from build123d import *

# Parameters (mm, degrees)
BOSS_EXTRUDE1_DEPTH      = 3.175
BOSS_EXTRUDE1_DEPTH_BACK = 19.05
SKETCH2_R                = 6.35
CUT_EXTRUDE1_DEPTH       = 41.348741461
CUT_EXTRUDE1_DEPTH_BACK  = 41.348741461
SKETCH3_R                = 0.79375
FILLET1_R                = 3.175
CHAMFER1_SIZE            = 1.27


with BuildPart() as part:
    # Sketch1 → Revolve1 (revolve)
    with BuildSketch(Plane.XY, mode=Mode.PRIVATE) as revolve1_sk:
        with BuildLine():
            Line((-1.5875, -19.05), (-1.5875, -23.8125))
            Line((-1.5875, -23.8125), (-3.175, -23.8125))
            Line((-3.175, -23.8125), (-3.175, 0))
            Line((-3.175, 0), (3.175, 0))
            Line((3.175, 0), (3.175, -23.8125))
            Line((3.175, -23.8125), (1.5875, -23.8125))
            Line((1.5875, -23.8125), (1.5875, -19.05))
            ThreePointArc((1.5875, -19.05), (0, -17.4625), (-1.5875, -19.05))
        make_face()
    revolve(revolve1_sk.sketch.rotate(Axis((-3.175, 0, 0), (1, 0, 0)), 270), axis=Axis((-3.175, 0, 0), (1, 0, 0)))

    # Sketch2 → Boss-Extrude1 (add, two sides: drawn at the far end of the back side and taken through both)
    with BuildSketch(Plane.ZY.offset(3.175).offset(-BOSS_EXTRUDE1_DEPTH_BACK)):
        Circle(SKETCH2_R)
    extrude(amount=BOSS_EXTRUDE1_DEPTH + BOSS_EXTRUDE1_DEPTH_BACK)

    # Sketch3 → Cut-Extrude1 (cut, two sides: drawn at the far end of the back side and taken through both)
    with BuildSketch(Plane.ZY.offset(6.35).offset(-CUT_EXTRUDE1_DEPTH_BACK)):
        Circle(SKETCH3_R)
    extrude(amount=CUT_EXTRUDE1_DEPTH + CUT_EXTRUDE1_DEPTH_BACK, mode=Mode.SUBTRACT)

    # Fillet1
    fillet1_edges = [part.edges().sort_by_distance(p)[0] for p in [
        (-3.175, 0, -6.35),
        (3.175, 0, -6.35),
    ]]
    fillet(fillet1_edges, radius=FILLET1_R - 0.0001)  # a hair under: the kernel refuses the full size

    # Chamfer1
    chamfer1_edges = [part.edges().sort_by_distance(p)[0] for p in [
        (-1.5875, 0, -23.8125),
        (1.5875, 0, -23.8125),
    ]]
    chamfer(chamfer1_edges, length=CHAMFER1_SIZE)


solid = part.part
The listing builds one solid part. Answer for the finished solid, in the listing's coordinates (mm). A direction names the side the tool comes from. Round coordinates to 2 decimals unless told otherwise and drop trailing zeros. Order: outer loops, then holes, each group sorted by start corner. A loop starts at its lowest first (then second) coordinate and runs counter-clockwise, first axis right, second up. Notation, with made-up numbers: (66.25, 63.5) -> (103.25, 63.5) arc R19 ccw to (103.25, 99.5) -> close; hole circle Ø1 at (56.5, 25). An arc over 180 degrees is marked (long way). Write each question's results on one line, items separated by ' | '. Start each with the question number.
Q1. Which of the six approach directions +Z, -Z, +X, -X, +Y, -Y give full straight-line access (tool end or side, diameter ignored) to faces 1 (the flat face through (1.587, -17, -10)), 2 (the flat face through (3.175, 0, -10)), 3 (the flat face through (15.875, 0, 1)), 4 (the flat face through (-3.175, 0, 10))?
Q2. Find section D-D (x = 5.5). Determine the outline of the cut face in (y, z).
Q3. The mould has two halves that part along Z. Classify faces 5 (the cylindrical face through (4.918, -0.775, -0.172)), 6 (the flat face through (-6.35, 0, 1)), 7 (the cylindrical face through (3.014, 23.246, -5.162)): pulls with the +Z half, pulls with the -Z half, needs draft (parallel to the pull), parting line crosses it, or undercut.
Q4. Straight lines are drawn through the part: probe 1 along Z at (x, y) = (11, 0); probe 2 along X at (y, z) = (-13.5, 14) (1 decimal). For each, find the intervals that lie inside material, in ascending order. Write a range as from..to.
Q5. Find section C-C (x = 10.25). Determine the outline of the cut face in (y, z).
Q6. Each of these flat-tipped pins is pushed along its axis until it touches: pin 1 (12 mm diameter, centred on y = -15, z = -10, fed in from +X) (3 decimals); pin 2 (3 mm diameter, centred on y = 14.5, z = 3.5, fed in from -X) (3 decimals); pin 3 (8 mm diameter, centred on x = 4.5, y = -10, fed in from -Z); pin 4 (1.3 mm diameter, centred on y = 0, z = 0, fed in from -X). Where does it stop, or does it pass through?
Worked answers:
1) face 1: none | face 2: +X | face 3: +Z, -Z, +X, +Y, -Y | face 4: -X
2) outline: circle Ø12.93 at (0, 0); hole circle Ø1.59 at (0, 0)
3) face 5: undercut | face 6: needs draft | face 7: parting line crosses it
4) probe 1: z = -6.35..-0.79, 0.79..6.35 | probe 2: x = -3.2..-1.6, 1.6..3.2
5) outline: circle Ø12.7 at (0, 0); hole circle Ø1.59 at (0, 0)
6) pin 1: stops at x = 3.175 | pin 2: stops at x = -3.175 | pin 3: stops at z = -22.98 | pin 4: passes through
